The drawing under review shows one solid part. Ordinate dimensions are in mm from its lowest x, y, z. A direction names the side the tool comes from. Coordinates: 2 decimals unless noted, no trailing zeros. Write each loop counter-clockwise with the first axis right and the second up, starting at its lowest first coordinate (ties: lowest second). Pieces come first, ordered by that corner, then holes. Notation, with made-up numbers: (-38, 38.25) -> (-34, 38.25) arc R26 ccw to (-34, 56.25) -> close; hole circle Ø8 at (34.5, -20). An arc over 180 degrees is marked (long way). One line per question, with ' | ' between items. Start each with the question number.
Q1. Add section D-D on y = 51. State the section outline as (x, z) points, and give its area (3 significant figures).
Q2. Add section A-A on y = 77. State the section outline as (x, z) points, and give its area (3 significant figures).
Q3. For P1, Ø2, axis at x = 96.5, z = 78, coming from the +Y side; P2, Ø4, axis at y = 25.5, z = 66, coming from the +X side; P3, Ø10, axis at y = 113.5, z = 127.5, coming from the -X side, all flat-tipped, find the tip position at first contact; note any pin that passes through.
Q4. Wall thickness on probe 1 along X at (y, z) = (115, 90); probe 2 along X at (y, z) = (109.5, 139); probe 3 along Y at (x, z) = (119, 77): over which ranges is each line inside the solid? List them lowest first.
Q5. Add section C-C on x = 24.5. State the section outline as (y, z) points.
Q6. For the marked faces 1, 2 and 3, list the 3-axis set-ups (+Z, -Z, +X, -X, +Y, -Y) from which the entire face can be reached by the end or side of a thin tool; tool diameter is ignored.
Q7. Draft analysis for pull direction X (two halves, no side actions). For the marked faces 4, 5, 6 and 7, state which applies: pulls with the +X half, pulls with the -X half, needs draft (parallel to the pull), parting line crosses it, or undercut.
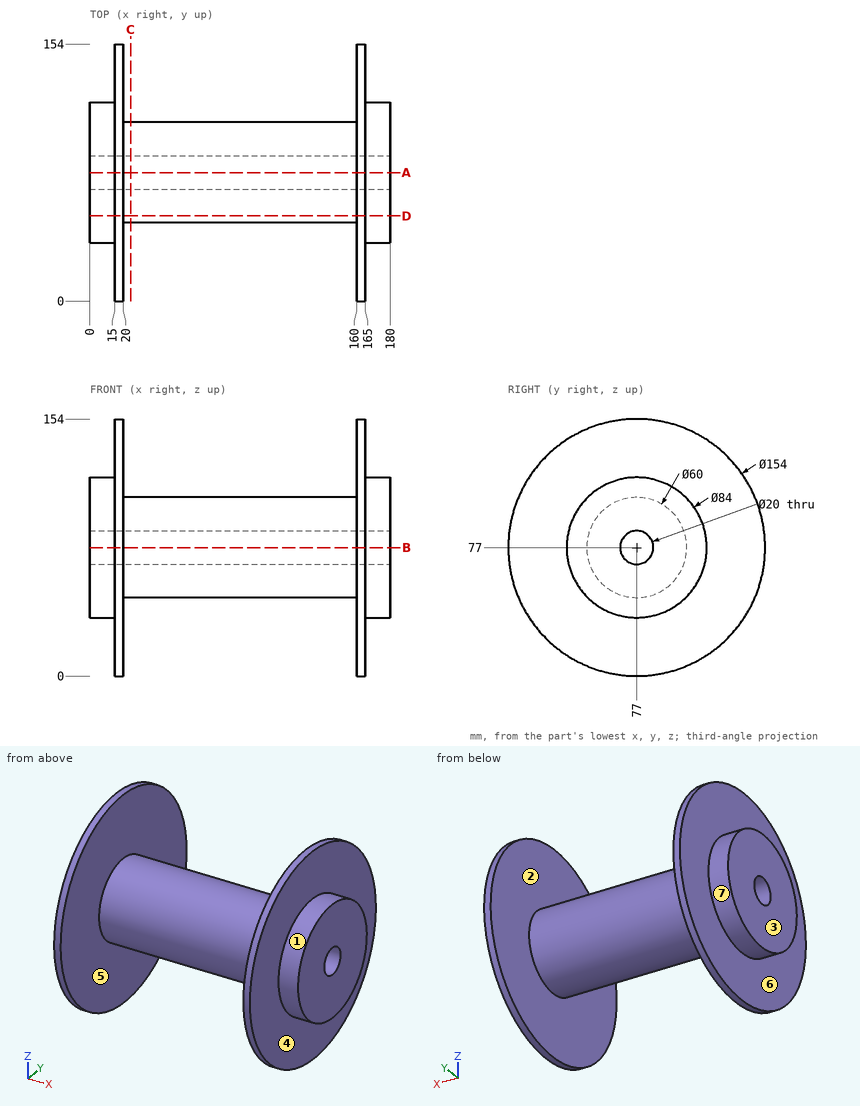
Output values:
1) outline: (0, 44.02) -> (15, 44.02) -> (15, 4.52) -> (20, 4.52) -> (20, 62.03) -> (160, 62.03) -> (160, 4.52) -> (165, 4.52) -> (165, 44.02) -> (180, 44.02) -> (180, 109.98) -> (165, 109.98) -> (165, 149.48) -> (160, 149.48) -> (160, 91.97) -> (20, 91.97) -> (20, 149.48) -> (15, 149.48) -> (15, 109.98) -> (0, 109.98) -> close | area: 7,620 mm2
2) outline: (0, 35) -> (15, 35) -> (15, 0) -> (20, 0) -> (20, 47) -> (160, 47) -> (160, 0) -> (165, 0) -> (165, 35) -> (180, 35) -> (180, 67) -> (0, 67) -> close; (0, 87) -> (180, 87) -> (180, 119) -> (165, 119) -> (165, 154) -> (160, 154) -> (160, 107) -> (20, 107) -> (20, 154) -> (15, 154) -> (15, 119) -> (0, 119) -> close | area: 8,860 mm2
3) P1: stops at y = 107 | P2: stops at x = 165 | P3: stops at x = 15
4) probe 1: x = 0 to 20, 160 to 180 | probe 2: x = 15 to 20, 160 to 165 | probe 3: y = 47 to 67, 87 to 107
5) outline: circle Ø60 at (77, 77); hole circle Ø20 at (77, 77)
6) face 1: +X | face 2: none | face 3: +Z, -Z, -X, +Y, -Y
7) face 4: pulls with the +X half | face 5: undercut | face 6: pulls with the -X half | face 7: needs draft
